Design review of the part built by this model. Coordinates are the model's own, in mm. A direction names the side the tool comes from. Round coordinates to 2 decimals unless told otherwise and drop trailing zeros. Write each loop counter-clockwise with the first axis right and the second up, starting at its lowest first coordinate (ties: lowest second). Pieces come first, ordered by that corner, then holes.
from build123d import *

# Parameters (mm, degrees)
SKETCH1_R           = 3.25
BOSS_EXTRUDE1_DEPTH = 10
SKETCH2_R           = 1.75
CUT_EXTRUDE1_DEPTH  = 2.5
SKETCH3_W           = 12.7
SKETCH3_H           = 7.4168
BOSS_EXTRUDE2_DEPTH = 5
FILLET1_R           = 2.54


with BuildPart() as part:
    # Sketch1 → Boss-Extrude1 (new body)
    with BuildSketch(Plane(origin=(0, 0, 0), x_dir=(1, 0, 0), z_dir=(0, 1, 0))):
        Circle(SKETCH1_R)
    extrude(amount=BOSS_EXTRUDE1_DEPTH)

    # Sketch2 → Cut-Extrude1 (cut)
    with BuildSketch(Plane.XZ):
        Circle(SKETCH2_R)
    extrude(amount=-CUT_EXTRUDE1_DEPTH, mode=Mode.SUBTRACT)

    # Sketch3 → Boss-Extrude2 (add)
    with BuildSketch(Plane(origin=(0, 10, 0), x_dir=(1, 0, 0), z_dir=(0, 1, 0))):
        Rectangle(SKETCH3_W, SKETCH3_H)
    extrude(amount=BOSS_EXTRUDE2_DEPTH)

    # Fillet1
    fillet1_edges = [part.edges().sort_by_distance(p)[0] for p in [
        (6.35, 12.5, 3.7084),
        (6.35, 12.5, -3.7084),
        (-6.35, 12.5, -3.7084),
        (-6.35, 12.5, 3.7084),
    ]]
    fillet(fillet1_edges, radius=FILLET1_R)


solid = part.part
1) For line 1 along Z through (x, y) = (0, 0.85); line 2 along Y through (x, z) = (1, 3.5); line 3 along Y through (x, z) = (-1.25, 0.25), list the stretches that pass through material, from the lowest coordinate up.
2) For P1, Ø3, axis at x = -2.5, y = 4.5, coming from the -Z side; P2, Ø3, axis at x = -4, y = 2, coming from the -Z side, all flat-tipped, find the tip position at first contact; note any pin that passes through.
3) Add section C-C on y = 12. State the section outline as (x, z) points, and give its area (3 significant figures).
4) Add section D-D on y = 1.5. State the section outline as (x, z) points.
5) Add section B-B on x = 0. State the section outline as (y, z) points, and give its area (3 significant figures).
6) For faces 1 (the face through (-2.579, 4.93, 1.978)), 2 (the face through (5.59, 12.54, -2.98)), list the 3-axis set-ups (+Z, -Z, +X, -X, +Y, -Y) from which the entire face can be reached by the end or side of a thin tool; tool diameter is ignored.
7) Add section A-A on z = 0. State the section outline as (x, y) points.
Computed:
1. line 1: z = -3.25 to -1.75, 1.75 to 3.25
1. line 2: y = 10 to 15
1. line 3: y = 2.5 to 15
2. P1: stops at z = -3.09
2. P2: stops at z = -2.08
3. outline: (-6.35, -1.17) arc R2.54 ccw to (-3.81, -3.71) - (3.81, -3.71) arc R2.54 ccw to (6.35, -1.17) - (6.35, 1.17) arc R2.54 ccw to (3.81, 3.71) - (-3.81, 3.71) arc R2.54 ccw to (-6.35, 1.17) - close
3. area: 88.7 mm2
4. outline: circle Ø6.5 at (0, 0); hole circle Ø3.5 at (0, 0)
5. outline: (0, -3.25) - (10, -3.25) - (10, -3.71) - (15, -3.71) - (15, 3.71) - (10, 3.71) - (10, 3.25) - (0, 3.25) - (0, 1.75) - (2.5, 1.75) - (2.5, -1.75) - (0, -1.75) - close
5. area: 93.3 mm2
6. face 1: -Y
6. face 2: -Z, +X, +Y, -Y
7. outline: (-6.35, 10) - (-3.25, 10) - (-3.25, 0) - (-1.75, 0) - (-1.75, 2.5) - (1.75, 2.5) - (1.75, 0) - (3.25, 0) - (3.25, 10) - (6.35, 10) - (6.35, 15) - (-6.35, 15) - close
